Verification items for this drawing (mm, ordinates from the low corner). A direction names the side the tool comes from. Coordinates: 2 decimals unless noted, no trailing zeros. Order: outer loops, then holes, each group sorted by start corner. A loop starts at its lowest first (then second) coordinate and runs counter-clockwise, first axis right, second up. Notation, with made-up numbers: (56.5, 58.25) -> (112.5, 58.25) arc R25 cw to (112.5, 72.25) -> close; hole circle Ø6 at (41, 34.25). An arc over 180 degrees is marked (long way). Put each result on its own line as item: value. Start each with the question number.
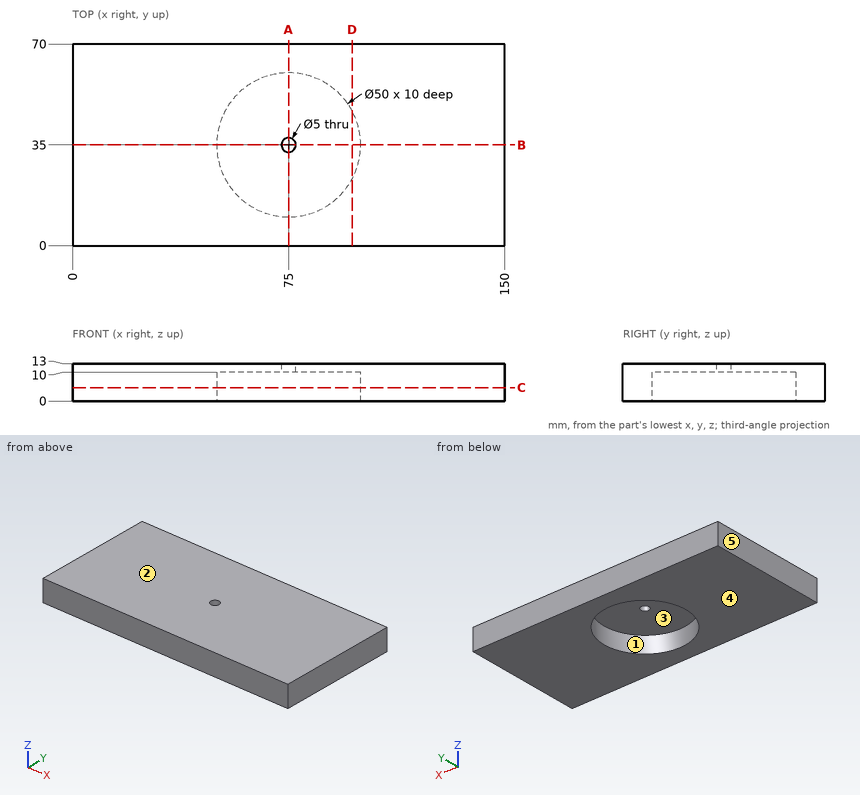
1) Sectioned sample at A-A (x = 75). Record the boundary of the cut face in (y, z).
2) Scan lines: line 1 along Y through (x, z) = (75, 12.25); line 2 along Y through (x, z) = (75, 7.5); line 3 along Z through (x, y) = (74.5, 42). Record each from-to range of solid material in increasing order. Write a range as [from, to].
3) Gauge pin test, flat end, axial feed: pin 1 (15 mm diameter, centred on x = 73, y = 34.5, fed in from -Z). Record the tip position at first contact, or that the pin passes through.
4) Sectioned sample at B-B (y = 35). Record the boundary of the cut face in (x, z), plus the area to 4 significant figures.
5) Sectioned sample at D-D (x = 97). Record the boundary of the cut face in (y, z), plus the area to 3 significant figures.
6) Access from +Z, -Z, +X, -X, +Y, -Y to the whole of each face (thin tool, end or side, straight path). Record for the marked faces 1 and 2.
7) Mould release check, pull along X, two halves, no side actions. Record for the marked faces 3, 4 and 5: +X half, -X half, draft (parallel to the pull), parting line (faces both ways), or undercut.
8) Sectioned sample at C-C (z = 4.75). Record the boundary of the cut face in (x, y).
Entries:
1. outline: (0, 0) -> (10, 0) -> (10, 10) -> (32.5, 10) -> (32.5, 13) -> (0, 13) -> close; (37.5, 10) -> (60, 10) -> (60, 0) -> (70, 0) -> (70, 13) -> (37.5, 13) -> close
2. line 1: y = [0, 32.5], [37.5, 70]
2. line 2: y = [0, 10], [60, 70]
2. line 3: z = [10, 13]
3. pin 1: stops at z = 10
4. outline: (0, 0) -> (50, 0) -> (50, 10) -> (72.5, 10) -> (72.5, 13) -> (0, 13) -> close; (77.5, 10) -> (100, 10) -> (100, 0) -> (150, 0) -> (150, 13) -> (77.5, 13) -> close
4. area: 1,435 mm2
5. outline: (0, 0) -> (23.13, 0) -> (23.13, 10) -> (46.87, 10) -> (46.87, 0) -> (70, 0) -> (70, 13) -> (0, 13) -> close
5. area: 673 mm2
6. face 1: -Z
6. face 2: +Z, +X, -X, +Y, -Y
7. face 3: undercut
7. face 4: draft
7. face 5: -X half
8. outline: (0, 0) -> (150, 0) -> (150, 70) -> (0, 70) -> close; hole circle Ø50 at (75, 35)
